from build123d import *

# Parameters (mm, degrees)
EXTRUDE_1_DEPTH        = 828.5
SKETCH_2_R             = 3.5
CUT_EXTRUDE_1_DEPTH    = 829.979794687
CUT_EXTRUDE_2_DEPTH    = 830.895324725
CUT_EXTRUDE_3_DEPTH    = 10
PATTERN_LINEAR_1_COUNT = 12
PATTERN_LINEAR_1_PITCH = 140


with BuildPart() as part:
    # Эскиз1 → Бобышка-Вытянуть1 (new, symmetric)
    with BuildSketch(Plane.XY):
        Polygon((22.5, 0), (-22.5, 0), (-22.5, 10.4), (-7.5, 10.4), (-7.5, 17), (7.5, 17), (7.5, 10.4), (22.5, 10.4), align=None)
    extrude(amount=EXTRUDE_1_DEPTH, both=True)

    # Эскиз2 → Вырез-Вытянуть1 (cut, through all)
    with BuildSketch(Plane(origin=(0, 17, 0), x_dir=(1, 0, 0), z_dir=(0, 1, 0))):
        with Locations(Location((0, -778.5, 0), (0, 0, 270))):
            Circle(SKETCH_2_R)
        with Locations(Location((0, -638.5, 0), (0, 0, 270))):
            Circle(SKETCH_2_R)
        with Locations(Location((0, -498.5, 0), (0, 0, 270))):
            Circle(SKETCH_2_R)
        with Locations(Location((0, -358.5, 0), (0, 0, 270))):
            Circle(SKETCH_2_R)
        with Locations(Location((0, -218.5, 0), (0, 0, 270))):
            Circle(SKETCH_2_R)
        with Locations(Location((0, -78.5, 0), (0, 0, 270))):
            Circle(SKETCH_2_R)
        with Locations(Location((0, 61.5, 0), (0, 0, 270))):
            Circle(SKETCH_2_R)
        with Locations(Location((0, 201.5, 0), (0, 0, 270))):
            Circle(SKETCH_2_R)
        with Locations(Location((0, 341.5, 0), (0, 0, 270))):
            Circle(SKETCH_2_R)
        with Locations(Location((0, 481.5, 0), (0, 0, 270))):
            Circle(SKETCH_2_R)
    extrude(amount=-CUT_EXTRUDE_1_DEPTH, mode=Mode.SUBTRACT)

    # Эскиз5 → Вырез-Вытянуть2 (cut, through all)
    with BuildSketch(Plane(origin=(22.5, 0, 0), x_dir=(0, 0, -1), z_dir=(1, 0, 0))):
        Polygon((-828.5, 0), (-811.5, 17), (-828.5, 17), align=None)
        Polygon((828.5, 17), (828.5, 0), (811.5, 17), align=None)
    extrude(amount=-CUT_EXTRUDE_2_DEPTH, mode=Mode.SUBTRACT)

    # Эскиз6 → Вырез-Вытянуть3 (cut)
    with BuildSketch(Plane(origin=(0, 17, 0), x_dir=(1, 0, 0), z_dir=(0, 1, 0))):
        with BuildLine():
            Line((-5, -775.613248654), (-5, -781.386751346))
            ThreePointArc((-5, -781.386751346), (0, -786.386751346), (5, -781.386751346))
            Line((5, -781.386751346), (5, -775.613248654))
            ThreePointArc((5, -775.613248654), (0, -770.613248654), (-5, -775.613248654))
        make_face()
    cut_extrude_3 = extrude(amount=-CUT_EXTRUDE_3_DEPTH, mode=Mode.SUBTRACT)

    # Линейный массив1: Вырез-Вытянуть3 ×12
    with Locations(*[(0, 0, -i * PATTERN_LINEAR_1_PITCH) for i in range(1, PATTERN_LINEAR_1_COUNT)]):
        add(cut_extrude_3, mode=Mode.SUBTRACT)


solid = part.part
Here's how the part is built. I have some questions about the finished solid (model axes, mm). Round coordinates to 2 decimals unless told otherwise and drop trailing zeros. Order: outer loops, then holes, each group sorted by start corner. A loop starts at its lowest first (then second) coordinate and runs counter-clockwise, first axis right, second up. Notation, with made-up numbers: M 70.5,15.25 L 110.5,15.25 A31 cw 110.5,50.25 Z; hole C -9,2 d4. An arc over 180 degrees is marked long. One line per question, with ' | ' between items.
1) I need wall thicknesses on line 1 (X direction, y = 4.5, z = 358.5); line 2 (X direction, y = 14.5, z = 359); line 3 (Y direction, x = 10, z = 726). Which ranges of each line are inside material? Lowest first, please.
Checked values:
line 1: x = -22.5 to -3.5, 3.5 to 22.5 | line 2: x = -7.5 to -5, 5 to 7.5 | line 3: y = 0 to 10.4
2) Imagine slicing it at A-A, the plane z = -428.5. Write out the boundary of the cut face in (x, y), plus the area to 3 significant figures.
Checked values:
outline: M -22.5,0 L 22.5,0 L 22.5,10.4 L 7.5,10.4 L 7.5,17 L -7.5,17 L -7.5,10.4 L -22.5,10.4 Z | area: 567 mm²
3) Imagine slicing it at B-B, the plane y = 14. Count the separate pieces of the cut face and the enclosed holes in it, plus the area to 3 significant figures.
Checked values:
separate pieces: 1 | enclosed holes: 12 | area: 22,800 mm²
4) I'm going to push flat-ended pins straight in: pin 1 Ø1.5 at (x, y) = (17.5, 5) entering from +Z; pin 2 Ø2 at (x, y) = (12.5, 7.5) entering from +Z; pin 3 Ø4 at (x, y) = (2, 4.5) entering from -Z. Where does each tip first touch, or does it pass through?
Checked values:
pin 1: stops at z = 824.25 | pin 2: stops at z = 822 | pin 3: stops at z = -826
